```python
from build123d import *

# Parameters (mm, degrees)
BOSS_EXTRUDE1_DEPTH      = 304.8
BOSS_EXTRUDE1_DEPTH_BACK = 304.8
CHAMFER1_SIZE            = 0.254
SKETCH5_R                = 12.7
SKETCH5_R_2              = 9.525
CUT_EXTRUDE1_DEPTH       = 458.55264178
SKETCH6_W                = 6
SKETCH6_H                = 6
CUT_EXTRUDE2_DEPTH       = 458.55264178
CHAMFER2_SIZE            = 0.2
SKETCH7_R                = 63.5
CUT_EXTRUDE3_DEPTH       = 357.053282529


with BuildPart() as part:
    # Sketch3 → Boss-Extrude1 (new, two sides: drawn at the far end of the back side and taken through both)
    with BuildSketch(Plane.XY.offset(-BOSS_EXTRUDE1_DEPTH_BACK)):
        with BuildLine():
            Line((-3.175, 9.525), (-3.175, 12.296722124))
            ThreePointArc((-3.175, 12.296722124), (0, -12.7), (3.175, 12.296722124))
            Line((3.175, 12.296722124), (3.175, 9.525))
            Line((3.175, 9.525), (-3.175, 9.525))
        make_face()
    extrude(amount=BOSS_EXTRUDE1_DEPTH + BOSS_EXTRUDE1_DEPTH_BACK)

    # Chamfer1
    chamfer1_edges = [part.edges().sort_by_distance(p)[0] for p in [
        (0, -12.7, -304.8),
        (0, -12.7, 304.8),
    ]]
    chamfer(chamfer1_edges, length=CHAMFER1_SIZE)

    # Sketch5 → Cut-Extrude1 (cut, through all)
    with BuildSketch(Plane.XY.offset(152.4)):
        Circle(SKETCH5_R)
        Circle(SKETCH5_R_2, mode=Mode.SUBTRACT)
    extrude(amount=-CUT_EXTRUDE1_DEPTH, mode=Mode.SUBTRACT)

    # Sketch6 → Cut-Extrude2 (cut, through all)
    with BuildSketch(Plane.XY.offset(152.4)):
        with Locations((0, 9.525)):
            Rectangle(SKETCH6_W, SKETCH6_H)
    extrude(amount=-CUT_EXTRUDE2_DEPTH, mode=Mode.SUBTRACT)

    # Chamfer2
    chamfer2_edges = [part.edges().sort_by_distance(p)[0] for p in [
        (-3.175, 10.910861062, 152.4),
        (0, -12.7, 152.4),
        (3.175, 10.910861062, 152.4),
        (0, 9.525, 152.4),
        (0, -9.525, 152.4),
        (-3, 7.782611309, 152.4),
        (0, 6.525, 152.4),
        (3, 7.782611309, 152.4),
    ]]
    chamfer(chamfer2_edges, length=CHAMFER2_SIZE)

    # Sketch7 → Cut-Extrude3 (cut, through all)
    with BuildSketch(Plane.XY.offset(50.8)):
        Circle(SKETCH7_R)
    extrude(amount=-CUT_EXTRUDE3_DEPTH, mode=Mode.SUBTRACT)


solid = part.part
```
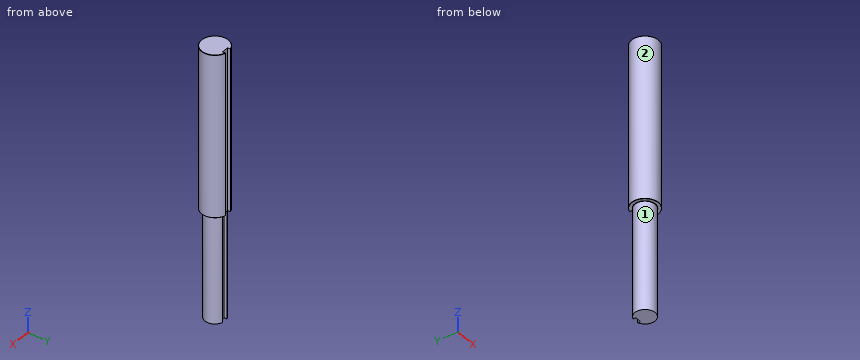
Can you work these out from the model? Positions are in its coordinate system, mm. Face numbers are marked on the shaded views. A direction names the side the tool comes from. Coordinates: 2 decimals unless noted, no trailing zeros. Loops run counter-clockwise (first coordinate to the right, second up) from the corner with the lowest first, then second, coordinate; pieces in that order, holes last. Notation, with made-up numbers: (-13.5, -31) - (33.5, -31) arc R10 ccw to (33.5, -22) - close; hole circle Ø11 at (-23, -8.75). An arc over 180 degrees is marked (long way). Answer as CSV lines item,"result". Start each with the question number.
1) Which directions (+Z, -Z, +X, -X, +Y, -Y) give clear straight access to the entire face, cutting with the end or side of a thin tool? Please do the marked faces 1 and 2.
2) I need wall thicknesses on line 1 (Z direction, x = -4.25, y = 10.5); line 2 (Y direction, x = -0.5, z = 184) (3 decimals); line 3 (X direction, y = 7.75, z = 125). Which ranges of each line are inside material? Lowest first, please. Write a range as from..to.
3) For pin 1 (2 mm diameter, centred on y = -6.5, z = 187.5, fed in from +X); pin 2 (1.5 mm diameter, centred on y = 2.5, z = 184, fed in from +X); pin 3 (0.8 mm diameter, centred on y = 10.5, z = 252.5, fed in from +X), each with a flat end and sliding along its axis, tell me the tip position at first contact or that it passes through.
4) Suppose I cut it at C-C (z = 112.5). Please give me the cut outline in (x, y) (3 decimals), plus the area to 3 significant figures.
5) Suppose I cut it at A-A (y = 0). Please give me the cut outline in (x, z) (3 decimals), plus the area to 3 significant figures.
6) Suppose I cut it at B-B (x = 0). Please give me the cut outline in (y, z) (3 decimals), plus the area to 3 significant figures.
Check result:
1,face 1,"-Z"
1,face 2,"+Z, -Z"
2,line 1,"z = 152.4..304.8"
2,line 2,"y = -12.69..9.525"
2,line 3,"x = -5.54..-3, 3..5.54"
3,pin 1,"stops at x = 11.45"
3,pin 2,"stops at x = 12.58"
3,pin 3,"stops at x = 7.7"
4,outline,"(-3, 6.525) - (-3, 9.04) arc R9.525 ccw (long way) to (3, 9.04) - (3, 6.525) - close"
4,area,"268 mm²"
5,outline,"(-12.7, 152.6) - (-12.5, 152.4) - (-9.725, 152.4) - (-9.525, 152.2) - (-9.525, 50.8) - (9.525, 50.8) - (9.525, 152.2) - (9.725, 152.4) - (12.5, 152.4) - (12.7, 152.6) - (12.7, 304.546) - (12.446, 304.8) - (-12.446, 304.8) - (-12.7, 304.546) - close"
5,area,"5,810 mm²"
6,outline,"(-12.7, 152.6) - (-12.5, 152.4) - (-9.725, 152.4) - (-9.525, 152.2) - (-9.525, 50.8) - (6.525, 50.8) - (6.525, 152.2) - (6.725, 152.4) - (9.325, 152.4) - (9.525, 152.6) - (9.525, 304.8) - (-12.446, 304.8) - (-12.7, 304.546) - close"
6,area,"5,020 mm²"
